The figure shows three views and two pictorial views of one solid part (mm, origin at its lowest corner). Answer the questions. A direction names the side the tool comes from. Round coordinates to 2 decimals unless told otherwise and drop trailing zeros. Write each loop counter-clockwise with the first axis right and the second up, starting at its lowest first coordinate (ties: lowest second). Pieces come first, ordered by that corner, then holes.
Item 1: Find the intervals of material crossed by probe 1 along Z at (x, y) = (20, 16.95); probe 2 along Z at (x, y) = (20, 8.5); probe 3 along Y at (x, z) = (4, 8.5), in increasing order.
Item 2: Each of these flat-tipped pins is pushed along its axis until it touches: pin 1 (2 mm diameter, centred on y = 16, z = 5, fed in from +X); pin 2 (2 mm diameter, centred on x = 18, z = 15.5, fed in from -Y); pin 3 (12 mm diameter, centred on y = 7, z = 6, fed in from -X); pin 4 (12 mm diameter, centred on x = 29, z = 17.5, fed in from -Y). Where does it stop, or does it pass through?
Item 3: Find section D-D on x = 30. Give the vertices of the cut face in (y, z), then the cut area to 3 significant figures.
Item 4: Find section B-B on z = 20. Give the vertices of the cut face in (x, y), then the cut area to 3 significant figures.
Item 5: For a pull along X with two mould halves and no side action, classify the marked faces 3, 4 and 5 as +X half, -X half, draft (parallel to the pull), parting line (faces both ways), or undercut.
Item 6: Find section A-A on x = 20. Give the vertices of the cut face in (y, z).
Item 7: Find section C-C on z = 31. Give the vertices of the cut face in (x, y).
Item 8: A tool of negligible diameter and unlimited length cuts with its end or side. For the marked faces 1 and 2, from which of +Z, -Z, +X, -X, +Y, -Y can it reach the whole face along a straight path? Write none if from no direction.
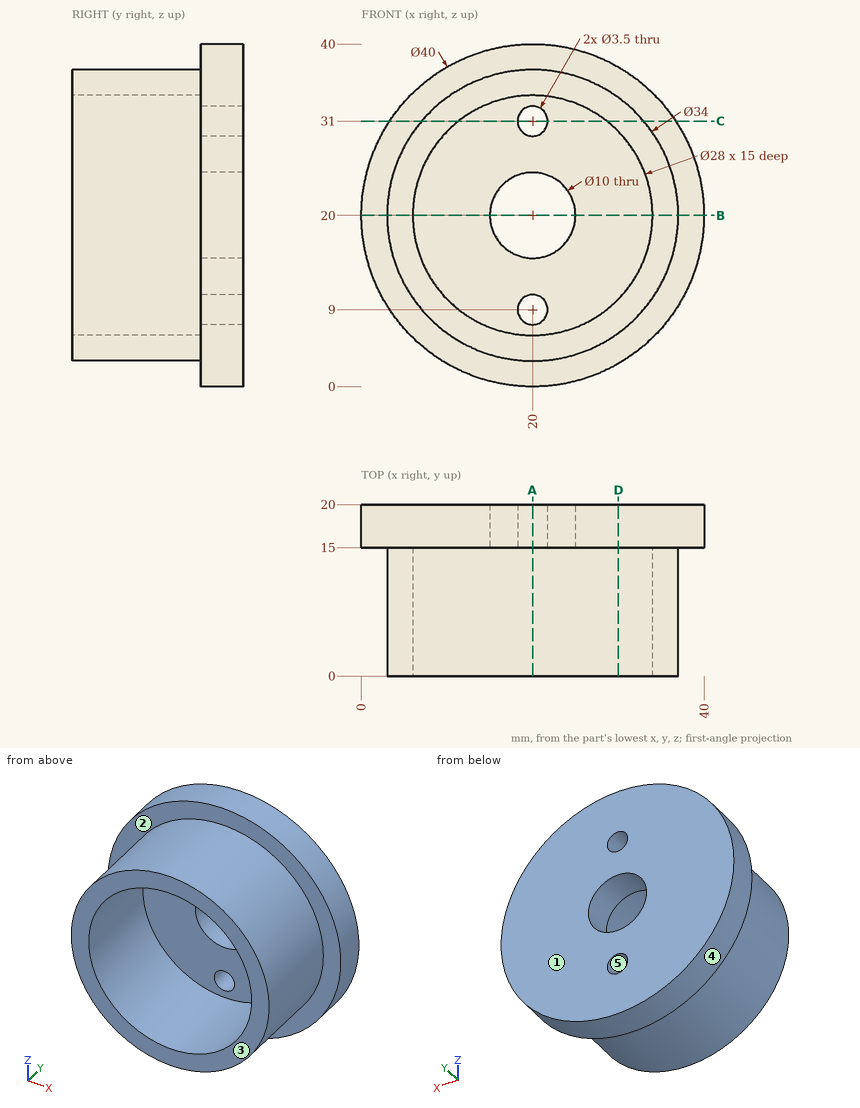
Check values:
1. probe 1: z = 0 to 7.25, 10.75 to 15, 25 to 29.25, 32.75 to 40
1. probe 2: z = 3 to 6, 34 to 37
1. probe 3: y = 15 to 20
2. pin 1: stops at x = 34.28
2. pin 2: stops at y = 15
2. pin 3: stops at x = 5
2. pin 4: stops at y = 0
3. outline: (0, 6.25) - (15, 6.25) - (15, 2.68) - (20, 2.68) - (20, 37.32) - (15, 37.32) - (15, 33.75) - (0, 33.75) - (0, 29.8) - (15, 29.8) - (15, 10.2) - (0, 10.2) - close
3. area: 292 mm2
4. outline: (0, 15) - (3, 15) - (3, 0) - (6, 0) - (6, 15) - (15, 15) - (15, 20) - (0, 20) - close; (25, 15) - (34, 15) - (34, 0) - (37, 0) - (37, 15) - (40, 15) - (40, 20) - (25, 20) - close
4. area: 240 mm2
5. face 3: draft
5. face 4: parting line
5. face 5: undercut
6. outline: (0, 3) - (15, 3) - (15, 0) - (20, 0) - (20, 7.25) - (15, 7.25) - (15, 6) - (0, 6) - close; (0, 34) - (15, 34) - (15, 32.75) - (20, 32.75) - (20, 40) - (15, 40) - (15, 37) - (0, 37) - close; (15, 10.75) - (20, 10.75) - (20, 15) - (15, 15) - close; (15, 25) - (20, 25) - (20, 29.25) - (15, 29.25) - close
7. outline: (3.3, 15) - (7.04, 15) - (7.04, 0) - (11.34, 0) - (11.34, 15) - (18.25, 15) - (18.25, 20) - (3.3, 20) - close; (21.75, 15) - (28.66, 15) - (28.66, 0) - (32.96, 0) - (32.96, 15) - (36.7, 15) - (36.7, 20) - (21.75, 20) - close
8. face 1: +Z, -Z, +X, -X, +Y
8. face 2: -Y
